Source: CAD feature listing. Evaluate the final solid. Frame: model axes, mm. A direction names the side the tool comes from. Give positions to 0.01 mm unless a question says otherwise; leave off trailing zeros. Write each loop counter-clockwise with the first axis right and the second up, starting at its lowest first coordinate (ties: lowest second). Pieces come first, ordered by that corner, then holes. Notation, with made-up numbers: (-20.5, 32.25) - (-9.5, 32.25) arc R14 cw to (-9.5, 49.25) - close; hole circle Ø9 at (2.5, 14). An arc over 180 degrees is marked (long way). One line per question, with ' | ' between items. Start each with the question number.
(1) Section B-B, the plane z = 0. State how many separate pieces and enclosed holes the cut face has, plus the area to 3 significant figures.
(2) Ray query, line 1 (Z direction, x = 4, y = 1.5); line 2 (X direction, y = 2.4, z = 26). Return the intervals inside material, ascending. Write a range as [from, to].
(3) Draft query along Z for faces 6 (the cylindrical face through (-11.9, 2.5, -0.5)), 7 (the cylindrical face through (-0.1, 1.7, 42.5)), 8 (the flat face through (-37.4, 1.5, 1.4)), 9 (the cylindrical face through (13.52, 1.73, -38.89)). Return one class per face: +Z half, -Z half, draft (parallel to the pull), parting line (faces both ways), or undercut.
(4) Section A-A, the plane z = 21. Return loops of the section in (x, y), plus the area to 4 significant figures.
(5) Pin query (flat end, axial travel): pin 1 (1.9 mm diameter, centred on x = 0, z = -9.76, fed in from +Y); pin 2 (1.8 mm diameter, centred on x = 25.5, y = 2, fed in from -Z); pin 3 (2 mm diameter, centred on x = -9.5, z = 0, fed in from +Y); pin 4 (1 mm diameter, centred on y = 1, z = -3, fed in from +X). Return the tip coordinate at first contact, or that it passes through.
(6) Access query for faces 1 (the cylindrical face through (0.1, 1.7, -42.5)), 2 (the flat face through (-15, 2, 25)), 3 (the flat face through (-15, 2, -25)), 4 (the flat face through (-12.409, 2, 0)), 5 (the flat face through (-1.4, 1.5, -9.8)). Directions: +Z, -Z, +X, -X, +Y, -Y. A direction counts if a zero-diameter tool reaches every point of the face in a straight line with its end or side. Return the directions, or none.
```python
from build123d import *

# Parameters (mm, degrees)
SKETCH_1_R                   = 42.5
SKETCH_1_W                   = 12.5
SKETCH_1_H                   = 22.4
SKETCH_1_W_2                 = 22.4
SKETCH_1_H_2                 = 12.5
EXTRUDE_1_DEPTH              = 3.5
HOLE_WIZARD_M2_1_D           = 2.4
HOLE_WIZARD_M2_1_CBORE_D     = 4.4
HOLE_WIZARD_M2_1_CBORE_DEPTH = 2
SKETCH_5_W                   = 28.893914533
SKETCH_5_H                   = 29.378378832
SKETCH_5_W_2                 = 29.378378832
SKETCH_5_H_2                 = 28.893914533
CUT_EXTRUDE_1_DEPTH          = 10
FILLET_1_R                   = 7


with BuildPart() as part:
    # 草图1 → 凸台-拉伸1 (new body)
    with BuildSketch(Plane(origin=(0, 0, 0), x_dir=(1, 0, 0), z_dir=(0, 1, 0))):
        with Locations(Location((0, 0, 0), (0, 0, 270))):
            Circle(SKETCH_1_R)
        with Locations((0, 23.608701573)):
            Rectangle(SKETCH_1_W, SKETCH_1_H, mode=Mode.SUBTRACT)
        with Locations((-23.608701573, 0)):
            Rectangle(SKETCH_1_W_2, SKETCH_1_H_2, mode=Mode.SUBTRACT)
        with Locations((23.608701573, 0)):
            Rectangle(SKETCH_1_W_2, SKETCH_1_H_2, mode=Mode.SUBTRACT)
        with Locations((0, -23.608701573)):
            Rectangle(SKETCH_1_W, SKETCH_1_H, mode=Mode.SUBTRACT)
    extrude(amount=EXTRUDE_1_DEPTH)

    # M2 凹头盖螺钉的柱形沉头孔1 (through all)
    with Locations(Plane(origin=(-9.758701573, 3.5, 0), x_dir=(0, 0, 1), z_dir=(0, 1, 0))):
        with Locations((0, 0), (-9.758701573, 9.758701573), (0, 19.517403146), (9.758701573, 9.758701573), (0, 47.217403146), (-37.458701573, 9.758701573), (0, -27.7), (37.458701573, 9.758701573)):
            CounterBoreHole(HOLE_WIZARD_M2_1_D / 2, HOLE_WIZARD_M2_1_CBORE_D / 2, HOLE_WIZARD_M2_1_CBORE_DEPTH)

    # 草图5 → 切除-拉伸1 (cut)
    with BuildSketch(Plane(origin=(0, 3.5, 0), x_dir=(1, 0, 0), z_dir=(0, 1, 0))):
        with Locations((29.446957267, 29.689189416)):
            Rectangle(SKETCH_5_W, SKETCH_5_H)
        with Locations((-29.689189416, 29.446957267)):
            Rectangle(SKETCH_5_W_2, SKETCH_5_H_2)
        with Locations((29.689189416, -29.446957267)):
            Rectangle(SKETCH_5_W_2, SKETCH_5_H_2)
        with Locations((-29.446957267, -29.689189416)):
            Rectangle(SKETCH_5_W, SKETCH_5_H)
    extrude(amount=-CUT_EXTRUDE_1_DEPTH, mode=Mode.SUBTRACT)

    # 圆角1
    fillet_1_edges = [part.edges().sort_by_distance(p)[0] for p in [
        (-39.764934301, 1.75, -15),
        (-15, 1.75, -39.764934301),
        (-39.764934301, 1.75, 15),
        (-15, 1.75, 39.764934301),
        (15, 1.75, 39.764934301),
        (39.764934301, 1.75, 15),
        (39.764934301, 1.75, -15),
        (15, 1.75, -39.764934301),
    ]]
    fillet(fillet_1_edges, radius=FILLET_1_R)


solid = part.part
```
Check sheet entries:
1) separate pieces: 7 | enclosed holes: 0 | area: 91.1 mm²
2) line 1: [-42.31, -34.81], [-12.41, 12.41], [34.81, 42.31] | line 2: [-15, -6.25], [6.25, 15]
3) face 6: undercut | face 7: +Z half | face 8: undercut | face 9: -Z half
4) outline: (-15, 0) - (-6.25, 0) - (-6.25, 3.5) - (-15, 3.5) - close; (6.25, 0) - (15, 0) - (15, 3.5) - (6.25, 3.5) - close | area: 61.25 mm²
5) pin 1: through | pin 2: z = -15 | pin 3: y = 1.5 | pin 4: x = 42.43
6) face 1: -Z, +Y, -Y | face 2: +Z, -X, +Y, -Y | face 3: -Z, -X, +Y, -Y | face 4: +Y, -Y | face 5: +Y
